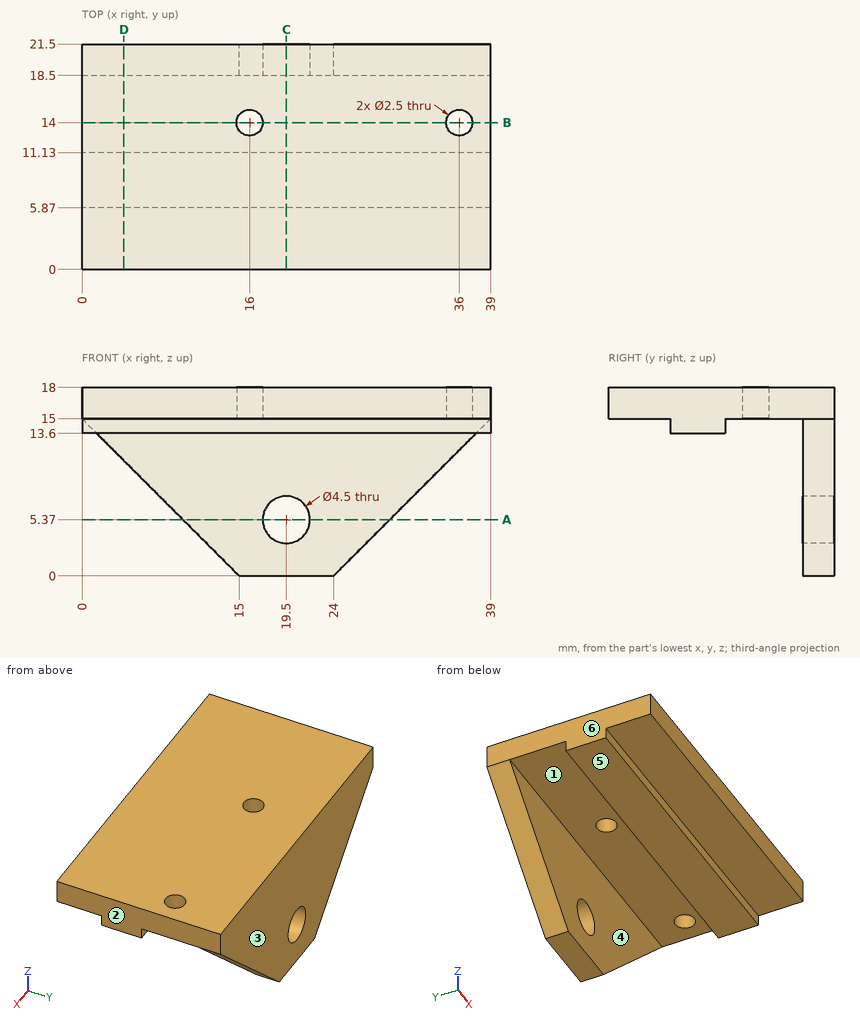
Design review of the part shown in the three views and the two pictorial views. Dimensions are in mm from the part's minimum x, y and z. A direction names the side the tool comes from. Round coordinates to 2 decimals unless told otherwise and drop trailing zeros. Loops run counter-clockwise (first coordinate to the right, second up) from the corner with the lowest first, then second, coordinate; pieces in that order, holes last.
Q1. Add section C-C on x = 19.5. Write out the cut boundary in (y, z), plus the area to 3 significant figures.
Result sheet:
outline: (0, 15) - (5.87, 15) - (5.87, 13.6) - (11.13, 13.6) - (11.13, 15) - (18.5, 15) - (18.5, 7.62) - (21.5, 7.62) - (21.5, 18) - (0, 18) - close; (18.5, 0) - (21.5, 0) - (21.5, 3.12) - (18.5, 3.12) - close
area: 103 mm2
Q2. Add section B-B on y = 14. Write out the cut boundary in (x, z), plus the area to 3 significant figures.
Result sheet:
outline: (0, 15) - (14.75, 15) - (14.75, 18) - (0, 18) - close; (17.25, 15) - (34.75, 15) - (34.75, 18) - (17.25, 18) - close; (37.25, 15) - (39, 15) - (39, 18) - (37.25, 18) - close
area: 102 mm2
Q3. Add section A-A on z = 5.37. Write out the cut boundary in (x, y).
Result sheet:
outline: (9.63, 18.5) - (17.25, 18.5) - (17.25, 21.5) - (9.63, 21.5) - close; (21.75, 18.5) - (29.37, 18.5) - (29.37, 21.5) - (21.75, 21.5) - close
Q4. Insertion check: pin 1 Ø1 at (y, z) = (17.5, 6) entering from +X; pin 2 Ø2.5 at (x, y) = (28, 8) entering from -Z; pin 3 Ø1.5 at (x, z) = (25, 14) entering from -Y; pin 4 Ø3 at (x, z) = (26.5, 3) entering from -Y. Each pin has a flat end and moves straight along its axis. Give the tip position at first contact, or say it passes through.
Result sheet:
pin 1: passes through
pin 2: stops at z = 13.6
pin 3: stops at y = 5.87
pin 4: stops at y = 18.5
Q5. Mouldability with a two-part tool opening along Y and no side actions: class the marked faces 1, 2 and 3 as +Y half, -Y half, draft (parallel to the pull), parting line (faces both ways), or undercut.
Result sheet:
face 1: undercut
face 2: draft
face 3: +Y half
Q6. Machinability: for the marked faces 4, 5 and 6, which of the approach directions +Z, -Z, +X, -X, +Y, -Y give a long, thin tool a straight path to every point of the face, cutting with its end or side? Answer none if there is none.
Result sheet:
face 4: -Z, +X, -X
face 5: -Z, +X, -X, -Y
face 6: +Z, -Z, -X, +Y, -Y
Q7. Add section D-D on x = 4. Write out the cut boundary in (y, z), plus the area to 3 significant figures.
Result sheet:
outline: (0, 15) - (5.87, 15) - (5.87, 13.6) - (11.13, 13.6) - (11.13, 15) - (18.5, 15) - (18.5, 11) - (21.5, 11) - (21.5, 18) - (0, 18) - close
area: 83.9 mm2
Q8. To check wall thickness, follow line 1 along Y through (x, z) = (16.5, 14.75); line 2 along Z through (x, y) = (19.5, 19.95); line 3 along Y through (x, z) = (36, 15.9). State the ranges of each line that lie inside material, in increasing order.
Result sheet:
line 1: y = 5.87 to 11.13, 18.5 to 21.5
line 2: z = 0 to 3.12, 7.62 to 18
line 3: y = 0 to 12.75, 15.25 to 21.5
